Can you work these out from the model? Positions are in its coordinate system, mm. Face numbers are marked on the shaded views. Coordinates: 2 decimals unless noted, no trailing zeros. Write each loop counter-clockwise with the first axis right and the second up, starting at its lowest first coordinate (ties: lowest second). Pieces come first, ordered by that corner, then holes. Notation, with made-up numbers: (51, 31) - (83, 31) arc R22 cw to (83, 43) - close; hole circle Ø4 at (75.25, 0.25). An arc over 180 degrees is marked (long way). Use one line per item in the form item = value. Start each with the question number.
(1) If we section it at A-A on x = -13.5: Please give me the cut outline in (y, z).
(2) For pin 1 Ø3 at (x, z) = (-9, 49.5) entering from +Y; pin 2 Ø8 at (y, z) = (9.5, 6) entering from +X; pin 3 Ø7 at (x, z) = (3, 15.5) entering from +Y, each with a flat end and sliding along its axis, tell me the tip position at first contact or that it passes through.
(3) If we section it at D-D on y = 14: Please give me the cut outline in (x, z) (3 decimals).
(4) If we section it at C-C on z = -68.5: Please give me the cut outline in (x, y), then the cut area to 3 significant figures.
(5) If I drill on probe 1 along X at (y, z) = (0.5, -68.5); probe 2 along X at (y, z) = (0.5, -87.5); probe 3 along Z at (x, y) = (2, 8), over which ranges is the centre line in solid material (lowest first)? Write a range as from..to.
(6) Thinking about a two-plate mould opening in Z: for the marked faces 1 and 2, which applies, pulls with the +Z half, pulls with the -Z half, needs draft (parallel to the pull), parting line crosses it, or undercut?
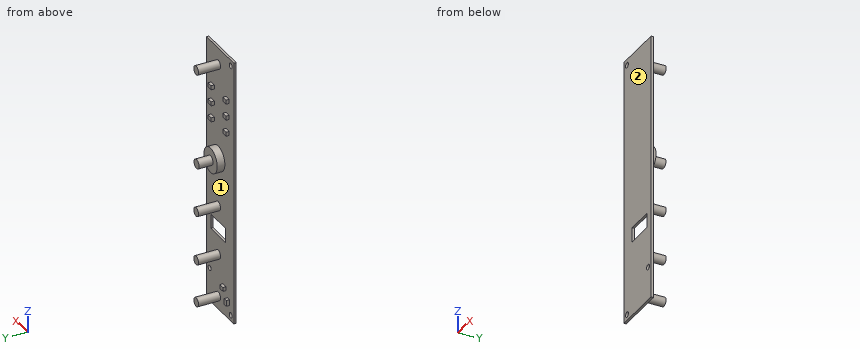
```python
from build123d import *

# Parameters (mm, degrees)
PCB_W               = 35
PCB_H               = 183
BOSS_EXTRUDE1_DEPTH = 1.6
SKETCH3_R           = 3
BOSS_EXTRUDE2_DEPTH = 15
SKETCH4_R           = 8.5
BOSS_EXTRUDE3_DEPTH = 5.21
SKETCH5_R           = 3.175
BOSS_EXTRUDE4_DEPTH = 9.52
SKETCH6_W           = 4
SKETCH6_H           = 2.9
BOSS_EXTRUDE5_DEPTH = 2.1
SKETCH7_R           = 1.85
CUT_EXTRUDE2_DEPTH  = 95.35835946
SKETCH8_W           = 4
SKETCH8_H           = 2.7
SKETCH8_W_2         = 2.7
SKETCH8_H_2         = 4
BOSS_EXTRUDE6_DEPTH = 2.1
SKETCH9_W           = 19
SKETCH9_H           = 10
CUT_EXTRUDE3_DEPTH  = 95.35835946


with BuildPart() as part:
    # pcb → Boss-Extrude1 (new body)
    with BuildSketch(Plane(origin=(0, 0, 0), x_dir=(1, 0, 0), z_dir=(0, 1, 0))):
        Rectangle(PCB_W, PCB_H)
    extrude(amount=BOSS_EXTRUDE1_DEPTH)

    # Sketch3 → Boss-Extrude2 (add)
    with BuildSketch(Plane(origin=(0, 1.6, 0), x_dir=(1, 0, 0), z_dir=(0, 1, 0))):
        with Locations(Location((2.5, 82.5, 0), (0, 0, 270))):
            Circle(SKETCH3_R)
        with Locations(Location((2.5, 53.25, 0), (0, 0, 270))):
            Circle(SKETCH3_R)
        with Locations(Location((2.5, 19.25, 0), (0, 0, 270))):
            Circle(SKETCH3_R)
        with Locations(Location((2.5, -80, 0), (0, 0, 270))):
            Circle(SKETCH3_R)
    extrude(amount=BOSS_EXTRUDE2_DEPTH)

    # Sketch4 → Boss-Extrude3 (add)
    with BuildSketch(Plane(origin=(0, 1.6, 0), x_dir=(1, 0, 0), z_dir=(0, 1, 0))):
        with Locations(Location((2.5, -14.25, 0), (0, 0, 270))):
            Circle(SKETCH4_R)
    extrude(amount=BOSS_EXTRUDE3_DEPTH)

    # Sketch5 → Boss-Extrude4 (add)
    with BuildSketch(Plane(origin=(0, 6.81, 0), x_dir=(1, 0, 0), z_dir=(0, 1, 0))):
        with Locations(Location((2.5, -14.25, 0), (0, 0, 270))):
            Circle(SKETCH5_R)
    extrude(amount=BOSS_EXTRUDE4_DEPTH)

    # Sketch6 → Boss-Extrude5 (add)
    with BuildSketch(Plane(origin=(0, 1.6, 0), x_dir=(1, 0, 0), z_dir=(0, 1, 0))):
        with Locations((-9.5, -39)):
            Rectangle(SKETCH6_W, SKETCH6_H)
        with Locations((9.5, -39)):
            Rectangle(SKETCH6_W, SKETCH6_H)
        with Locations((-9.5, -50.25)):
            Rectangle(SKETCH6_W, SKETCH6_H)
        with Locations((9.5, -50.25)):
            Rectangle(SKETCH6_W, SKETCH6_H)
        with Locations((-9.5, -61.5)):
            Rectangle(SKETCH6_W, SKETCH6_H)
        with Locations((9.5, -61.5)):
            Rectangle(SKETCH6_W, SKETCH6_H)
    extrude(amount=BOSS_EXTRUDE5_DEPTH)

    # Sketch7 → Cut-Extrude2 (cut, through all)
    with BuildSketch(Plane(origin=(0, 1.6, 0), x_dir=(1, 0, 0), z_dir=(0, 1, 0))):
        with Locations(Location((13.5, 68.5, 0), (0, 0, 270))):
            Circle(SKETCH7_R)
        with Locations(Location((-13.5, 87.5, 0), (0, 0, 270))):
            Circle(SKETCH7_R)
        with Locations(Location((-13.5, -87.5, 0), (0, 0, 270))):
            Circle(SKETCH7_R)
    extrude(amount=-CUT_EXTRUDE2_DEPTH, mode=Mode.SUBTRACT)

    # Sketch8 → Boss-Extrude6 (add)
    with BuildSketch(Plane(origin=(0, 1.6, 0), x_dir=(1, 0, 0), z_dir=(0, 1, 0))):
        with Locations((-5.5, 72)):
            Rectangle(SKETCH8_W, SKETCH8_H)
        with Locations((-10.5, 79.5)):
            Rectangle(SKETCH8_W_2, SKETCH8_H_2)
    extrude(amount=BOSS_EXTRUDE6_DEPTH)

    # Sketch9 → Cut-Extrude3 (cut, through all)
    with BuildSketch(Plane(origin=(0, 1.6, 0), x_dir=(1, 0, 0), z_dir=(0, 1, 0))):
        with Locations((2.5, 35)):
            Rectangle(SKETCH9_W, SKETCH9_H)
    extrude(amount=-CUT_EXTRUDE3_DEPTH, mode=Mode.SUBTRACT)


solid = part.part
```
Reported:
q1.outline = (0, -91.5) - (1.6, -91.5) - (1.6, -89.35) - (0, -89.35) - close; (0, -85.65) - (1.6, -85.65) - (1.6, 85.65) - (0, 85.65) - close; (0, 89.35) - (1.6, 89.35) - (1.6, 91.5) - (0, 91.5) - close
q2.pin_1 = 3.7
q2.pin_2 = 9.15
q2.pin_3 = 16.33
q3.outline = circle Ø6.35 at (2.5, 14.25); circle Ø6 at (2.5, -82.5); circle Ø6 at (2.5, -53.25); circle Ø6 at (2.5, -19.25); circle Ø6 at (2.5, 80)
q4.outline = (-17.5, 0) - (11.65, 0) - (11.65, 1.6) - (-17.5, 1.6) - close; (15.35, 0) - (17.5, 0) - (17.5, 1.6) - (15.35, 1.6) - close
q4.area = 50.1 mm2
q5.probe_1 = -17.5..11.65, 15.35..17.5
q5.probe_2 = -17.5..-15.35, -11.65..17.5
q5.probe_3 = -85.46..-79.54, -56.21..-50.29, -22.21..-16.29, 11.11..17.39, 77.04..82.96
q6.face_1 = undercut
q6.face_2 = needs draft
